```python
from build123d import *

# Parameters (mm, degrees)
F0_R     = 3.25
F1_DEPTH = 34
F3_DEPTH = 25
F4_W     = 25
F4_H     = 3
F5_DEPTH = 25


with BuildPart() as f1:
    # F0 (on Top) → F1 (new body)
    with BuildSketch(Plane.XY):
        with BuildLine():
            ThreePointArc((-29.961314, 5.041625), (-27.78708, 6.686189), (-26.961314, 9.284266))
            ThreePointArc((-26.961314, 9.284266), (-34.05939, 12.9585), (-32.961314, 5.041625))
            ThreePointArc((-32.961314, 5.041625), (-31.461314, 4.784266), (-29.961314, 5.041625))
        make_face()
        with Locations((-31.461314, 9.284266)):
            Circle(F0_R, mode=Mode.SUBTRACT)
        with BuildLine():
            ThreePointArc((-29.961314, 5.041625), (-31.461314, 4.784266), (-32.961314, 5.041625))
            Line((-32.961314, 5.041625), (-32.961314, -6.215734))
            Line((-32.961314, -6.215734), (2.038686, -6.215734))
            Line((2.038686, -6.215734), (2.038686, -4.965734))
            Line((2.038686, -4.965734), (-29.961314, -4.965734))
            Line((-29.961314, -4.965734), (-29.961314, 5.041625))
        make_face()
        with BuildLine():
            Line((2.038686, -6.215734), (-32.961314, -6.215734))
            Line((-32.961314, -6.215734), (-32.961314, -17.473094))
            ThreePointArc((-32.961314, -17.473094), (-31.461314, -17.215734), (-29.961314, -17.473094))
            Line((-29.961314, -17.473094), (-29.961314, -7.465734))
            Line((-29.961314, -7.465734), (2.038686, -7.465734))
            Line((2.038686, -7.465734), (2.038686, -6.215734))
        make_face()
        with BuildLine():
            ThreePointArc((-29.961314, -17.473094), (-31.461314, -17.215734), (-32.961314, -17.473094))
            ThreePointArc((-32.961314, -17.473094), (-34.05939, -25.389969), (-26.961314, -21.715734))
            ThreePointArc((-26.961314, -21.715734), (-27.78708, -19.117658), (-29.961314, -17.473094))
        make_face()
        with Locations((-31.461314, -21.715734)):
            Circle(F0_R, mode=Mode.SUBTRACT)
    extrude(amount=F1_DEPTH)

    # F2 (on face) → F3 (cut)
    with BuildSketch(Plane(origin=(-32.961314, 0, 0), x_dir=(0, -1, 0), z_dir=(-1, 0, 0))):
        with BuildLine():
            ThreePointArc((8.615734, 25.5), (12.715734, 21.4), (16.815734, 25.5))
            ThreePointArc((16.815734, 25.5), (12.715734, 29.6), (8.615734, 25.5))
        make_face()
    extrude(amount=-F3_DEPTH, mode=Mode.SUBTRACT)

    # F4 (on face) → F5 (cut)
    with BuildSketch(Plane.XZ.offset(7.465734)):
        with Locations((-12.5, 28.5)):
            Rectangle(F4_W, F4_H)
        with Locations((-12.5, 5.5)):
            Rectangle(F4_W, F4_H)
    extrude(amount=-F5_DEPTH, mode=Mode.SUBTRACT)


solid = f1.part
```
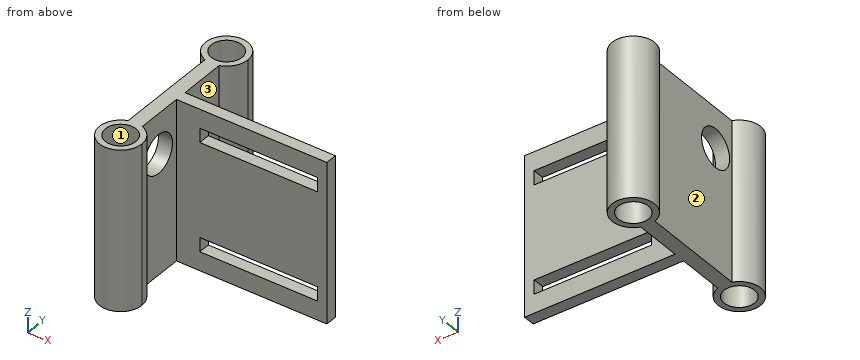
Part model, mm, in its own coordinate system. Face numbers are marked on the shaded views. A direction names the side the tool comes from. Round coordinates to 2 decimals unless told otherwise and drop trailing zeros. Write each loop counter-clockwise with the first axis right and the second up, starting at its lowest first coordinate (ties: lowest second). Pieces come first, ordered by that corner, then holes. Notation, with made-up numbers: (26.5, 24) -> (39.5, 24) arc R34 cw to (39.5, 60) -> close; hole circle Ø5 at (-19, -37). An arc over 180 degrees is marked (long way). Return JSON: item names as keys, results as strings. Group by question number.
Q1. Probe L1, parallel to Z at x = -24, y = -6; L2, parallel to Y at x = -31, z = 25; L3, parallel to X at y = -5, z = 27.5. List the from-to ranges inside material, lowest first. Write a range as [from, to].
Q2. Saw through at C-C on x = -19.5. Write the cut outline in (y, z), plus the area to 3 significant figures.
Q3. Which spindle directions (+Z, -Z, +X, -X, +Y, -Y) get a long thin tool onto all of the face, cutting with end or side? Do the marked faces 1, 2 and 3. Say none if no direction does.
Q4. Pin check, flat tips, straight feed: pin 1 (5 mm diameter, centred on x = -3.5, z = 17, fed in from -Y); pin 2 (2 mm diameter, centred on x = -28, z = 29.5, fed in from -Y); pin 3 (2 mm diameter, centred on x = -23.5, z = 23, fed in from +Y); pin 4 (10 mm diameter, centred on x = -15, y = 4, fed in from +Z). Stop position of each tip, or through.
Q5. Saw through at A-A on z = 25.5. Write the cut outline in (x, y), plus the area to 3 significant figures.
Q6. Saw through at B-B on y = -22.5. Write the cut outline in (x, z), plus the area to 3 significant figures.
Q7. Saw through at D-D on z = 20.5. Write the cut outline in (x, y).
Answer:
{
 "1": {"L1": "[0, 4], [7, 27], [30, 34]", "L2": "[-26.19, -24.93], [-18.5, -16.79], [-8.65, 6.07], [12.5, 13.76]", "L3": "[-32.96, -25], [0, 2.04]"},
 "2": {"outline": "(-7.47, 0) -> (-4.97, 0) -> (-4.97, 4) -> (-7.47, 4) -> close; (-7.47, 7) -> (-4.97, 7) -> (-4.97, 27) -> (-7.47, 27) -> close; (-7.47, 30) -> (-4.97, 30) -> (-4.97, 34) -> (-7.47, 34) -> close", "area": "70.0 mm2"},
 "3": {"face 1": "+Z, -Z", "face 2": "+Z, -Z, -X", "face 3": "+Z, -Z, +X"},
 "4": {"pin 1": "y = -7.47", "pin 2": "y = -25.48", "pin 3": "y = -4.97", "pin 4": "through"},
 "5": {"outline": "(-32.96, -17.47) arc R4.5 ccw (long way) to (-26.96, -21.72) arc R4.5 ccw to (-29.96, -17.47) -> (-29.96, -16.82) -> (-32.96, -16.82) -> close; (-32.96, -8.62) -> (-29.96, -8.62) -> (-29.96, -7.47) -> (2.04, -7.47) -> (2.04, -4.97) -> (-29.96, -4.97) -> (-29.96, 5.04) arc R4.5 ccw to (-26.96, 9.28) arc R4.5 ccw (long way) to (-32.96, 5.04) -> close; hole circle Ø6.5 at (-31.46, -21.72); hole circle Ø6.5 at (-31.46, 9.28)", "area": "183 mm2"},
 "6": {"outline": "(-35.89, 0) -> (-34.62, 0) -> (-34.62, 34) -> (-35.89, 34) -> close; (-28.31, 0) -> (-27.03, 0) -> (-27.03, 34) -> (-28.31, 34) -> close", "area": "86.8 mm2"},
 "7": {"outline": "(-32.96, -17.47) arc R4.5 ccw (long way) to (-26.96, -21.72) arc R4.5 ccw to (-29.96, -17.47) -> (-29.96, -7.47) -> (2.04, -7.47) -> (2.04, -4.97) -> (-29.96, -4.97) -> (-29.96, 5.04) arc R4.5 ccw to (-26.96, 9.28) arc R4.5 ccw (long way) to (-32.96, 5.04) -> close; hole circle Ø6.5 at (-31.46, -21.72); hole circle Ø6.5 at (-31.46, 9.28)"}
}
